CAD build for the part. Positions are in the model's coordinates, mm. A direction names the side the tool comes from. Round coordinates to 2 decimals unless told otherwise and drop trailing zeros. Order: outer loops, then holes, each group sorted by start corner. A loop starts at its lowest first (then second) coordinate and runs counter-clockwise, first axis right, second up. Notation, with made-up numbers: M -33.5,-34 L 18.5,-34 A19 ccw 18.5,-6 Z; hole C 21,64 d1. An arc over 180 degrees is marked long. Put each result on its own line as item: value.
```python
from build123d import *

# Parameters (mm, degrees)
F1_DEPTH = 63.5
F2_DEPTH = 25.4
F3_DEPTH = 7.9375


with BuildPart() as f1:
    # F0 (on Front) → F1 (new body, symmetric)
    with BuildSketch(Plane.XZ):
        Polygon((-41.275, 9.525), (-41.275, -9.525), (41.275, -9.525), (41.275, 9.525), (22.225, 9.525), align=None)
    extrude(amount=F1_DEPTH, both=True)

    # F0 (on Front) → F2 (join, symmetric)
    with BuildSketch(Plane.XZ):
        with BuildLine():
            Line((22.225, 9.525), (41.275, 9.525))
            Line((41.275, 9.525), (41.275, 27.0002))
            ThreePointArc((41.275, 27.0002), (45.92468, 38.22552), (57.15, 42.8752))
            Line((57.15, 42.8752), (60.325, 42.8752))
            Line((60.325, 42.8752), (60.325, 61.9252))
            Line((60.325, 61.9252), (57.15, 61.9252))
            ThreePointArc((57.15, 61.9252), (32.454296, 51.695904), (22.225, 27.0002))
            Line((22.225, 27.0002), (22.225, 9.525))
        make_face()
        Polygon((85.725, 61.9252), (60.325, 61.9252), (60.325, 42.8752), (60.325, 38.1), (85.725, 38.1), align=None)
    extrude(amount=F2_DEPTH, both=True)

    # F0 (on Front) → F3 (join, symmetric)
    with BuildSketch(Plane.XZ):
        with BuildLine():
            add(Edge.make_bspline(
                [(-41.275, 9.525), (0, 22.249181), (43.333913, 69.793309), (57.15, 61.9252)],
                knots=[0, 0, 0, 0, 111.504536, 111.504536, 111.504536, 111.504536], degree=3))
            Line((-41.275, 9.525), (22.225, 9.525))
            Line((22.225, 9.525), (22.225, 27.0002))
            ThreePointArc((22.225, 27.0002), (32.454296, 51.695904), (57.15, 61.9252))
        make_face()
    extrude(amount=F3_DEPTH, both=True)

    # F0 (on Front) → F4 (revolve)
    with BuildSketch(Plane.XZ):
        Polygon((85.725, 66.675), (85.725, 61.9252), (85.725, 38.1), (111.125, 38.1), (111.125, 66.675), align=None)
    revolve(axis=Axis((85.725, 0, 52.3875), (0, 0, 1)))


solid = f1.part
```
Item 1: Probe line 1 along Y through (x, z) = (-12.5, 22); line 2 along Z through (x, y) = (0.5, 45) (3 decimals); line 3 along X through (y, z) = (14, -2.5) (3 decimals). List the from-to ranges inside material, lowest first. Write a range as [from, to].
Answers below:
line 1: [-7.94, 7.94]
line 2: [-9.525, 9.525]
line 3: [-41.275, 41.275]
Item 2: Band-saw the part on A-A on y = 43. Give the cut face in (x, z) (3 decimals).
Answers below:
outline: M -41.275,-9.525 L 41.275,-9.525 L 41.275,9.525 L -41.275,9.525 Z
Item 3: Band-saw the part on B-B on x = 69. Give the cut face in (y, z) (3 decimals).
Answers below:
outline: M -25.4,38.1 L 25.4,38.1 L 25.4,61.925 L 19.116,61.925 L 19.116,66.675 L -19.116,66.675 L -19.116,61.925 L -25.4,61.925 Z
Item 4: Pin check, flat tips, straight feed: P1, Ø2, axis at x = 48, y = -2, coming from the +Z side; P2, Ø2.5, axis at x = 59.5, y = -4, coming from the -Z side; P3, Ø8.5, axis at y = 13.5, z = 14, coming from the -X side (3 decimals). Stop position of each tip, or through.
Answers below:
P1: z = 62.02
P2: z = 38.1
P3: x = 22.225
Item 5: Band-saw the part on C-C on y = 20.5. Give the cut face in (x, z) (3 decimals).
Answers below:
outline: M -41.275,-9.525 L 41.275,-9.525 L 41.275,27 A15.875 cw 57.15,42.875 L 60.325,42.875 L 60.325,38.1 L 100.722,38.1 L 100.722,66.675 L 70.728,66.675 L 70.728,61.925 L 57.15,61.925 A34.925 ccw 22.225,27 L 22.225,9.525 L -41.275,9.525 Z
Item 6: Mould opens along X. For faces 1 (the flat face through (-1, 63.5, 0)), 2 (the flat face through (60.325, 0, 41)), 3 (the flat face through (22.225, 17, 18)), 4 (the flat face through (41.275, -1, 4)) say: pulls with the +X half, pulls with the -X half, needs draft (parallel to the pull), parting line crosses it, or undercut.
Answers below:
face 1: needs draft
face 2: undercut
face 3: pulls with the -X half
face 4: pulls with the +X half
Item 7: Tool access for faces 5 (the cylindrical face through (45.8, -0.4, 38.1)), 6 (the flat face through (5, -7.938, 24)), 7 (the flat face through (5, 7.938, 24)), 8 (the cylindrical face through (109.95, 7.63, 55.76)), 9 (the flat face through (46, -25.4, 42)): list every direction of +Z, -Z, +X, -X, +Y, -Y with a clear straight run to the whole face (end or side of a thin tool).
Answers below:
face 5: -Z, +Y, -Y
face 6: +Z, -X, -Y
face 7: +Z, -X, +Y
face 8: +Z
face 9: +Z, +X, -X, -Y
